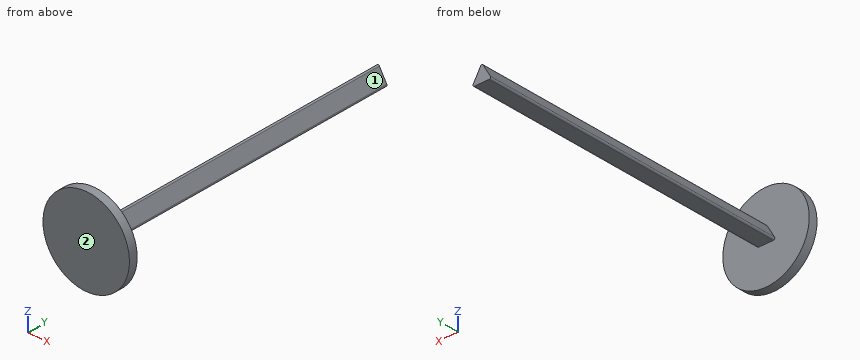
from build123d import *

# Parameters (mm, degrees)
SKETCH1_R           = 15.19
BOSS_EXTRUDE1_DEPTH = 3
BOSS_EXTRUDE2_DEPTH = 110


with BuildPart() as part:
    # Sketch1 → Boss-Extrude1 (new body)
    with BuildSketch(Plane(origin=(0, 0, 0), x_dir=(1, 0, 0), z_dir=(0, 1, 0))):
        with Locations(Location((0, 0, 0), (0, 0, 270))):
            Circle(SKETCH1_R)
    extrude(amount=BOSS_EXTRUDE1_DEPTH)

    # Sketch2 → Boss-Extrude2 (add)
    with BuildSketch(Plane(origin=(0, 3, 0), x_dir=(1, 0, 0), z_dir=(0, 1, 0))):
        with BuildLine():
            Line((0.433012702, -3.25), (3.031088913, 1.25))
            ThreePointArc((3.031088913, 1.25), (3.031088913, 1.75), (2.598076211, 2))
            Line((2.598076211, 2), (-2.598076211, 2))
            ThreePointArc((-2.598076211, 2), (-3.031088913, 1.75), (-3.031088913, 1.25))
            Line((-3.031088913, 1.25), (-0.433012702, -3.25))
            ThreePointArc((-0.433012702, -3.25), (0, -3.5), (0.433012702, -3.25))
        make_face()
    extrude(amount=BOSS_EXTRUDE2_DEPTH)


solid = part.part
CAD build for the part. Positions are in the model's coordinates, mm. Face numbers are marked on the shaded views. A direction names the side the tool comes from. Round coordinates to 2 decimals unless told otherwise and drop trailing zeros. Write each loop counter-clockwise with the first axis right and the second up, starting at its lowest first coordinate (ties: lowest second). Pieces come first, ordered by that corner, then holes. Notation, with made-up numbers: M -6,74.5 L 5,74.5 A11 ccw 5,95.5 Z; hole C 77,25 d11. An arc over 180 degrees is marked long. Use a Markdown table: item, result. Add a question column.
1. Slice it at A-A on y = 13. Give the cut face in (x, z).
2. Slice it at C-C on x = 11.5. Give the cut face in (y, z).
3. Slice it at B-B on z = 0. Give the cut face in (x, y).
4. Slice it at D-D on z = -10. Give the cut face in (x, y), then the cut area to 3 significant figures.
5. Flat gauge pins, fed straight in: P1, Ø2, axis at x = -4, y = 25, coming from the +Z side; P2, Ø1.5, axis at x = 9.5, z = 5.5, coming from the +Y side; P3, Ø15, axis at x = 7, z = 5.5, coming from the +Y side; P4, Ø4, axis at x = -1, y = 46.5, coming from the -Z side. Where does each tip first touch, or does it go through?
6. 3-axis set-ups, long thin cutter, end or side, ignore diameter. For the marked faces 1 and 2: which of +Z, -Z, +X, -X, +Y, -Y reach the whole face in a straight line?
7. Drill centre lines: probe 1 along Y at (x, z) = (7.5, 9); probe 2 along X at (y, z) = (62, -1.5); probe 3 along Z at (x, y) = (1, 57). Where is each one in solid material? Low to high.
Reply:
| question | item | result |
|---|---|---|
| 1 | outline | M -3.03,-1.25 A0.5 ccw -2.6,-2 L 2.6,-2 A0.5 ccw 3.03,-1.25 L 0.43,3.25 A0.5 ccw -0.43,3.25 Z |
| 2 | outline | M 0,-9.92 L 3,-9.92 L 3,9.92 L 0,9.92 Z |
| 3 | outline | M -15.19,0 L 15.19,0 L 15.19,3 L 2.31,3 L 2.31,113 L -2.31,113 L -2.31,3 L -15.19,3 Z |
| 4 | outline | M -11.43,0 L 11.43,0 L 11.43,3 L -11.43,3 Z |
| 4 | area | 68.6 mm^2 |
| 5 | P1 | stops at z = -1.2 |
| 5 | P2 | stops at y = 3 |
| 5 | P3 | stops at y = 113 |
| 5 | P4 | stops at z = -2 |
| 6 | face 1 | +Z, +X, +Y |
| 6 | face 2 | +Z, -Z, +X, -X, -Y |
| 7 | probe 1 | y = 0 to 3 |
| 7 | probe 2 | x = -3.1 to 3.1 |
| 7 | probe 3 | z = -2 to 2.27 |
